```python
from build123d import *

# Parameters (mm, degrees)
SKETCH1_R           = 50
SKETCH1_R_2         = 11.425
SKETCH1_R_3         = 1.45
BOSS_EXTRUDE1_DEPTH = 3
CUT_EXTRUDE4_REACH  = 72.774
CUT_EXTRUDE3_DEPTH  = 10


with BuildPart() as part:
    # Sketch1 → Boss-Extrude1 (new body)
    # profile 1 of 2: a face of its own
    with BuildSketch(Plane.XY):
        Circle(SKETCH1_R)
        Circle(SKETCH1_R_2, mode=Mode.SUBTRACT)
        with Locations((22.5, 38.97114317)):
            Circle(SKETCH1_R_3, mode=Mode.SUBTRACT)
        with Locations((-45, 0)):
            Circle(SKETCH1_R_3, mode=Mode.SUBTRACT)
        with Locations((22.5, -38.97114317)):
            Circle(SKETCH1_R_3, mode=Mode.SUBTRACT)
    # profile 2 of 2: a face of its own
    with BuildSketch(Plane.XY):
        with BuildLine():
            Line((-7.75, 35.822297768), (7.75, 35.822297768))
            ThreePointArc((7.75, 35.822297768), (10.898845402, 38.97114317), (7.75, 42.119988573))
            Line((7.75, 42.119988573), (-7.75, 42.119988573))
            ThreePointArc((-7.75, 42.119988573), (-10.898845402, 38.97114317), (-7.75, 35.822297768))
        make_face()
    extrude(amount=BOSS_EXTRUDE1_DEPTH)

    # Sketch1_6 → Cut-Extrude4 (cut, up to next)
    with BuildSketch(Plane.XY, mode=Mode.PRIVATE) as cut_extrude4_sk1:
        with BuildLine():
            Line((-7.75, 35.822297768), (7.75, 35.822297768))
            ThreePointArc((7.75, 35.822297768), (10.898845402, 38.97114317), (7.75, 42.119988573))
            Line((7.75, 42.119988573), (-7.75, 42.119988573))
            ThreePointArc((-7.75, 42.119988573), (-10.898845402, 38.97114317), (-7.75, 35.822297768))
        make_face()
    cut_extrude4_tool1 = extrude(cut_extrude4_sk1.sketch, amount=CUT_EXTRUDE4_REACH, mode=Mode.PRIVATE) & part.part
    add(cut_extrude4_tool1.solids().sort_by_distance((0, 38.971143, 0))[0], mode=Mode.SUBTRACT)

    # Sketch2 → Cut-Extrude3 (cut)
    with BuildSketch(Plane(origin=(0, 0, 0), x_dir=(-1, 0, 0), z_dir=(0, 0, -1))):
        with BuildLine():
            Line((-50.492676186, 4.91367638), (-33.753889757, 4.91367638))
            ThreePointArc((-33.753889757, 4.91367638), (-28.840213376, 0), (-33.753889757, -4.91367638))
            Line((-33.753889757, -4.91367638), (-50.492676186, -4.91367638))
            ThreePointArc((-50.492676186, -4.91367638), (-55.406352566, 0), (-50.492676186, 4.91367638))
        make_face()
        with BuildLine():
            Line((-34.573554166, 19), (-25.753889757, 19))
            ThreePointArc((-25.753889757, 19), (-24.253889757, 17.5), (-25.753889757, 16))
            Line((-25.753889757, 16), (-34.573554166, 16))
            ThreePointArc((-34.573554166, 16), (-36.073554166, 17.5), (-34.573554166, 19))
        make_face()
        with BuildLine():
            Line((-34.573554166, -19), (-25.753889757, -19))
            ThreePointArc((-25.753889757, -19), (-24.253889757, -17.5), (-25.753889757, -16))
            Line((-25.753889757, -16), (-34.573554166, -16))
            ThreePointArc((-34.573554166, -16), (-36.073554166, -17.5), (-34.573554166, -19))
        make_face()
    extrude(amount=-CUT_EXTRUDE3_DEPTH, mode=Mode.SUBTRACT)


solid = part.part
```
Geometry: final body of the model. Coordinates: model frame, mm. A direction names the side the tool comes from. Give positions to 0.01 mm unless a question says otherwise; leave off trailing zeros. Loops run counter-clockwise (first coordinate to the right, second up) from the corner with the lowest first, then second, coordinate; pieces in that order, holes last. Notation, with made-up numbers: (3, 74) -> (15, 74) arc R8 cw to (15, 85) -> close; hole circle Ø8 at (2.25, 80). An arc over 180 degrees is marked (long way). Return JSON: item names as keys, results as strings.
Item 1: Pin query (flat end, axial travel): P1, Ø1.7, axis at x = 22.5, y = -38.97, coming from the +Z side; P2, Ø1.5, axis at x = 38, z = 2, coming from the +Y side; P3, Ø0.9, axis at x = 41.5, z = 1.5, coming from the -Y side; P4, Ø1.5, axis at x = 32, z = 2, coming from the +Y side. Return the tip coordinate at first contact, or that it passes through.
Filled in:
{"P1": "through", "P2": "y = 33.35", "P3": "y = -28.55", "P4": "y = 39.03"}
Item 2: Line query: line 1 (Y direction, x = 22.5, z = 1); line 2 (Y direction, x = -9.5, z = 1.9); line 3 (Y direction, x = -45, z = 2). Output: solid intervals per line, ascending.
Filled in:
{"line 1": "-44.65 to -40.42, -37.52 to 37.52, 40.42 to 44.65", "line 2": "-49.09 to -6.35, 6.35 to 36.35, 41.59 to 49.09", "line 3": "-21.79 to -1.45, 1.45 to 21.79"}
Item 3: Section C-C, the plane x = -45. Output: boundary loops of the cut face in (y, z), plus the area to 3 significant figures.
Filled in:
{"outline": "(-21.79, 0) -> (-1.45, 0) -> (-1.45, 3) -> (-21.79, 3) -> close; (1.45, 0) -> (21.79, 0) -> (21.79, 3) -> (1.45, 3) -> close", "area": "122 mm^2"}
Item 4: Access query for faces 1 (the cylindrical face through (28.84, 0.11, 1.48)), 2 (the flat face through (0, 42.12, 1)). Directions: +Z, -Z, +X, -X, +Y, -Y. A direction counts if a zero-diameter tool reaches every point of the face in a straight line with its end or side. Return the directions, or none.
Filled in:
{"face 1": "+Z, -Z, +X", "face 2": "+Z, -Z"}
Item 5: Mould query, pull axis X, two halves, no side actions, for faces 3 (the cylindrical face through (23.2, 37.7, 1.5)), 4 (the cylindrical face through (-49.955, 2.13, 1.479)), 5 (the flat face through (-1, 12, 3)). Classes: released by +X, released by -X, zero draft, split by the parting line, or undercut.
Filled in:
{"face 3": "undercut", "face 4": "split by the parting line", "face 5": "zero draft"}
Item 6: Section D-D, the plane y = -17.5. Output: boundary loops of the cut face in (x, z).
Filled in:
{"outline": "(-46.84, 0) -> (24.25, 0) -> (24.25, 3) -> (-46.84, 3) -> close; (36.07, 0) -> (46.84, 0) -> (46.84, 3) -> (36.07, 3) -> close"}
Item 7: Section A-A, the plane x = 0. Output: boundary loops of the cut face in (y, z) (3 decimals), plus the area to 3 significant figures.
Filled in:
{"outline": "(-50, 0) -> (-11.425, 0) -> (-11.425, 3) -> (-50, 3) -> close; (11.425, 0) -> (35.822, 0) -> (35.822, 3) -> (11.425, 3) -> close; (42.12, 0) -> (50, 0) -> (50, 3) -> (42.12, 3) -> close", "area": "213 mm^2"}
Item 8: Section B-B, the plane z = 1.75. Output: boundary loops of the cut face in (x, y) (3 decimals).
Filled in:
{"outline": "(33.754, -4.914) arc R4.914 cw to (33.754, 4.914) -> (49.758, 4.914) arc R50 ccw (long way) to (49.758, -4.914) -> close; hole circle Ø2.9 at (-45, 0); hole circle Ø22.85 at (0, 0); hole (-7.75, 35.822) -> (7.75, 35.822) arc R3.149 ccw to (7.75, 42.12) -> (-7.75, 42.12) arc R3.149 ccw to start; hole circle Ø2.9 at (22.5, -38.971); hole circle Ø2.9 at (22.5, 38.971); hole (25.754, -19) -> (34.574, -19) arc R1.5 ccw to (34.574, -16) -> (25.754, -16) arc R1.5 ccw to start; hole (25.754, 16) -> (34.574, 16) arc R1.5 ccw to (34.574, 19) -> (25.754, 19) arc R1.5 ccw to start"}
